The listing builds one solid part. Answer for the finished solid, in the listing's coordinates (mm). A direction names the side the tool comes from. Round coordinates to 2 decimals unless told otherwise and drop trailing zeros. Loops run counter-clockwise (first coordinate to the right, second up) from the corner with the lowest first, then second, coordinate; pieces in that order, holes last. Notation, with made-up numbers: M 32,73 L 55,73 A24 ccw 55,89 Z; hole C 71,51 d2. An arc over 180 degrees is marked long. Answer as a JSON object with one key per item and string values.
```python
from build123d import *

# Parameters (mm, degrees)
SKETCH1_W               = 16
SKETCH1_H               = 87
BOSS_EXTRUDE2_DEPTH     = 12
CUT_EXTRUDE1_DEPTH      = 65.719189191
CUT_EXTRUDE1_DEPTH_BACK = 65.719189191
CUT_EXTRUDE2_DEPTH      = 65.719189191
CUT_EXTRUDE2_DEPTH_BACK = 65.719189191
SKETCH4_R               = 3
SKETCH4_R_2             = 1.5
BOSS_EXTRUDE3_DEPTH     = 2.5
FILLET1_R               = 1
FILLET2_R               = 10
SKETCH5_W               = 5
SKETCH5_H               = 10
SKETCH5_W_2             = 2.5
CUT_EXTRUDE3_DEPTH      = 5
CUT_EXTRUDE4_REACH      = 62.834
SKETCH6_W               = 5
SKETCH6_H               = 2.5
SKETCH7_W               = 5
SKETCH7_H               = 10
CUT_EXTRUDE5_DEPTH      = 65.719189191


with BuildPart() as part:
    # Sketch1 → Boss-Extrude2 (new body)
    with BuildSketch(Plane.XY):
        with Locations((0, -19.591785912)):
            Rectangle(SKETCH1_W, SKETCH1_H)
    extrude(amount=BOSS_EXTRUDE2_DEPTH)

    # Sketch2 → Cut-Extrude1 (cut, two sides: drawn at the far end of the back side and taken through both)
    with BuildSketch(Plane(origin=(0, 0, 0), x_dir=(0, 0, -1), z_dir=(1, 0, 0)).offset(-CUT_EXTRUDE1_DEPTH_BACK)):
        Polygon((0, 15.908214088), (0, 23.908214088), (-8, 23.908214088), align=None)
    extrude(amount=CUT_EXTRUDE1_DEPTH + CUT_EXTRUDE1_DEPTH_BACK, mode=Mode.SUBTRACT)

    # Sketch3 → Cut-Extrude2 (cut, two sides: drawn at the far end of the back side and taken through both)
    with BuildSketch(Plane(origin=(0, 0, 0), x_dir=(0, 0, -1), z_dir=(1, 0, 0)).offset(-CUT_EXTRUDE2_DEPTH_BACK)):
        with BuildLine():
            ThreePointArc((-3, 25.008214088), (-6.559834153, 27.955515518), (-8.791057147, 23.908214088))
            Line((-8.791057147, 23.908214088), (-7.019803903, 23.908214088))
            ThreePointArc((-7.019803903, 23.908214088), (-6.600122548, 26.382933306), (-4.5, 25.008214088))
            ThreePointArc((-4.5, 25.008214088), (-4.625280782, 24.40809154), (-4.980196097, 23.908214088))
            Line((-4.980196097, 23.908214088), (-3.208942853, 23.908214088))
            ThreePointArc((-3.208942853, 23.908214088), (-3.05269857, 24.448379935), (-3, 25.008214088))
        make_face()
        with BuildLine():
            Line((-7.019803903, 23.908214088), (-8.791057147, 23.908214088))
            ThreePointArc((-8.791057147, 23.908214088), (-6, 22.008214088), (-3.208942853, 23.908214088))
            Line((-3.208942853, 23.908214088), (-4.980196097, 23.908214088))
            ThreePointArc((-4.980196097, 23.908214088), (-6, 23.508214088), (-7.019803903, 23.908214088))
        make_face()
    extrude(amount=CUT_EXTRUDE2_DEPTH + CUT_EXTRUDE2_DEPTH_BACK, mode=Mode.SUBTRACT)

    # Sketch4 → Boss-Extrude3 (add, symmetric)
    with BuildSketch(Plane(origin=(0, 0, 0), x_dir=(0, 0, -1), z_dir=(1, 0, 0))):
        with Locations((-6, 25.008214088)):
            Circle(SKETCH4_R)
        with Locations((-6, 25.008214088)):
            Circle(SKETCH4_R_2, mode=Mode.SUBTRACT)
    extrude(amount=BOSS_EXTRUDE3_DEPTH, both=True)

    # Fillet1
    fillet1_edges = [part.edges().sort_by_distance(p)[0] for p in [
        (0, 22.009939252, 6.101725164),
        (0, 23.908214088, 8.791057147),
    ]]
    fillet(fillet1_edges, radius=FILLET1_R)

    # Fillet2
    fillet2_edges = [part.edges().sort_by_distance(p)[0] for p in [
        (0, 15.908214088, 0),
    ]]
    fillet(fillet2_edges, radius=FILLET2_R)

    # Sketch5 → Cut-Extrude3 (cut)
    with BuildSketch(Plane(origin=(0, 0, 0), x_dir=(-1, 0, 0), z_dir=(0, 0, -1))):
        with Locations((0, -16.091785912)):
            Rectangle(SKETCH5_W, SKETCH5_H)
        with Locations((1.25, -36.091785912)):
            Rectangle(SKETCH5_W_2, SKETCH5_H)
        with Locations((-1.25, -36.091785912)):
            Rectangle(SKETCH5_W_2, SKETCH5_H)
    extrude(amount=-CUT_EXTRUDE3_DEPTH, mode=Mode.SUBTRACT)

    # Sketch6 → Cut-Extrude4 (cut, up to next)
    with BuildSketch(Plane.XZ.offset(31.091785912), mode=Mode.PRIVATE) as cut_extrude4_sk1:
        with Locations((0, 3.75)):
            Rectangle(SKETCH6_W, SKETCH6_H)
    cut_extrude4_tool1 = extrude(cut_extrude4_sk1.sketch, amount=-CUT_EXTRUDE4_REACH, mode=Mode.PRIVATE) & part.part
    add(cut_extrude4_tool1.solids().sort_by_distance((0, -31.091786, 3.75))[0], mode=Mode.SUBTRACT)

    # Sketch7 → Cut-Extrude5 (cut, through all)
    with BuildSketch(Plane(origin=(0, 0, 0), x_dir=(-1, 0, 0), z_dir=(0, 0, -1))):
        with Locations((0, -36.091785912)):
            Rectangle(SKETCH7_W, SKETCH7_H)
    extrude(amount=-CUT_EXTRUDE5_DEPTH, mode=Mode.SUBTRACT)


solid = part.part
```
Item 1: Determine the mould class of faces 1 (the face through (-2.5, 23.6, 5)), 2 (the face through (0, -63.092, 6)), 3 (the face through (-2.5, -29.6, 4.6)), 4 (the face through (0, -41.092, 6)) for opening direction X: released by +X, released by -X, zero draft, split by the parting line, or undercut.
Values follow:
{"face 1": "released by -X", "face 2": "zero draft", "face 3": "undercut", "face 4": "undercut"}
Item 2: Flat-ended cylindrical pins translate along their axes: P1, Ø2.5, axis at x = 0.5, z = 10.5, coming from the +Y side; P2, Ø2.5, axis at y = 25.01, z = 6, coming from the -X side. Find the tip coordinate at first contact, or state that the pin passes through.
Values follow:
{"P1": "y = 24.25", "P2": "through"}
Item 3: The part is cut by section B-B (y = -19). Give the vertices of the cut face in (x, z).
Values follow:
{"outline": "M -8,0 L -2.5,0 L -2.5,5 L 2.5,5 L 2.5,0 L 8,0 L 8,12 L -8,12 Z"}
Item 4: Which of the six approach directions +Z, -Z, +X, -X, +Y, -Y give full straight-line access (tool end or side, diameter ignored) to faces 5 (the face through (0, -11.092, 2)), 6 (the face through (0, -31.092, 8)), 7 (the face through (2.5, 23.6, 5))?
Values follow:
{"face 5": "-Z", "face 6": "+Z, -Z", "face 7": "-Z, +X, +Y"}
Item 5: The part is cut by section A-A (x = -1). Give the vertices of the cut face in (y, z), then the cut area to 3 significant figures.
Values follow:
{"outline": "M -63.09,0 L -41.09,0 L -41.09,12 L -63.09,12 Z; M -31.09,0 L -21.09,0 L -21.09,2.5 L -31.09,2.5 Z; M -31.09,5 L -11.09,5 L -11.09,0 L 11.77,0 A10 ccw 18.84,2.93 L 20.76,4.85 A1 cw 22.35,4.61 A3 ccw long 24.93,9 A1 cw 23.91,10 L 23.91,12 L -31.09,12 Z; hole C 25.01,6 d3", "area": "835 mm^2"}
Item 6: Straight lines are drawn through the part: line 1 (Y direction, x = 0.45, z = 6); line 2 (Y direction, x = -0.5, z = 4.75); line 3 (X direction, y = -32, z = 11). For each, find the intervals that lie inside material, in ascending order.
Values follow:
{"line 1": "-63.09 to -41.09, -31.09 to 23.51, 26.51 to 28.01", "line 2": "-63.09 to -41.09, -11.09 to 20.66, 22.26 to 24.18, 25.84 to 27.74", "line 3": "-8 to -2.5, 2.5 to 8"}
